For this review, take the finished solid that the model builds, in its own axes (mm). A direction names the side the tool comes from. Round coordinates to 2 decimals unless told otherwise and drop trailing zeros. Order: outer loops, then holes, each group sorted by start corner. A loop starts at its lowest first (then second) coordinate and runs counter-clockwise, first axis right, second up. Notation, with made-up numbers: M 44,75 L 53,75 A26 cw 53,102 Z; hole C -10.75,-14.75 d7. An arc over 180 degrees is marked long. Answer as a JSON object with one key per item and string values.
from build123d import *

# Parameters (mm, degrees)
F0_R     = 9.5
F1_DEPTH = 225
F2_R     = 5.5
F3_DEPTH = 7
F4_SIZE  = 1
F5_R     = 8.5
F6_DEPTH = 20


with BuildPart() as f1:
    # F0 (on Front) → F1 (new body)
    with BuildSketch(Plane.XZ):
        Circle(F0_R)
    extrude(amount=F1_DEPTH)

    # F2 (on face) → F3 (join)
    with BuildSketch(Plane.XZ.offset(225)):
        Circle(F2_R)
    extrude(amount=F3_DEPTH)

    # F4
    f4_edges = [f1.edges().sort_by_distance(p)[0] for p in [
        (-5.5, -232, 0),
    ]]
    chamfer(f4_edges, length=F4_SIZE)

    # F5 (on face) → F6 (join)
    with BuildSketch(Plane(origin=(0, 0, 0), x_dir=(-1, 0, 0), z_dir=(0, 1, 0))):
        Circle(F5_R)
    extrude(amount=F6_DEPTH)

    # F7 (on Top) → F8 (revolve)
    with BuildSketch(Plane.XY):
        with BuildLine():
            Line((-8.5, 20), (0, 20))
            Line((0, 20), (0, 22))
            ThreePointArc((0, 22), (-4.366062, 21.493265), (-8.5, 20))
        make_face()
    revolve(axis=Axis((0, 10, 0), (0, -1, 0)))


solid = f1.part
1) Add section B-B on y = -116. State the section outline as (x, z) points.
Geometry check:
{"outline": "C 0,0 d19"}
2) For L1, parallel to X at y = -194, z = 4.25; L2, parallel to Y at x = -7.5, z = -5.5; L3, parallel to Y at x = 2, z = 4.5, list the stretches that pass through material, from the lowest coordinate up.
Geometry check:
{"L1": "x = -8.5 to 8.5", "L2": "y = -225 to 0", "L3": "y = -231.58 to 21.35"}
3) Insertion check: P1, Ø4, axis at x = -5, z = 4, coming from the +Y side; P2, Ø3, axis at x = -5.5, y = -98, coming from the -Z side; P3, Ø1, axis at y = -100, z = -6, coming from the -X side; P4, Ø4, axis at x = -1.5, y = -121.5, coming from the +Z side. Each pin has a flat end and moves straight along its axis. Give the tip position at first contact, or say it passes through.
Geometry check:
{"P1": "stops at y = 21.48", "P2": "stops at z = -8.62", "P3": "stops at x = -7.75", "P4": "stops at z = 9.5"}
4) Machinability: for faces 1 (the flat face through (0, -232, 0)), 2 (the flat face through (4, -225, -4)), 3 (the cylindrical face through (-4.57, 9.86, 7.167)), which of the approach directions +Z, -Z, +X, -X, +Y, -Y give a long, thin tool a straight path to every point of the face, cutting with its end or side? Answer none if there is none.
Geometry check:
{"face 1": "+Z, -Z, +X, -X, -Y", "face 2": "-Y", "face 3": "+Y"}
5) Add section A-A on y = 5. State the section outline as (x, z) points.
Geometry check:
{"outline": "C 0,0 d17"}
